Geometry: final body of the model. Coordinates: model frame, mm. Face numbers are marked on the shaded views. A direction names the side the tool comes from. Give positions to 0.01 mm unless a question says otherwise; leave off trailing zeros. Write each loop counter-clockwise with the first axis right and the second up, starting at its lowest first coordinate (ties: lowest second). Pieces come first, ordered by that corner, then holes. Notation, with made-up numbers: M 69.25,62 L 116.25,62 A30 cw 116.25,89 Z; hole C -21.5,39 d7. An arc over 180 degrees is marked long. Use one line per item in the form item = value. Start each with the question number.
Item 1: Pull-direction query (Y, two-part tool) for the marked faces 3, 4 and 5; classes: released by +Y, released by -Y, zero draft, split by the parting line, or undercut.
Item 2: Section query D-D on y = 507.5. Return loops of the section in (x, z), then the cut area to 3 significant figures.
Item 3: Section query A-A on z = -66.5. Return loops of the section in (x, y), then the cut area to 3 significant figures.
Item 4: Section query C-C on z = -90. Return loops of the section in (x, y), then the cut area to 3 significant figures.
Item 5: Contact query for flat-ended pins moving along their axis: P1, Ø2, axis at x = 14, z = -89, coming from the +Y side; P2, Ø6, axis at x = -17.5, z = -187.5, coming from the -Y side; P3, Ø3, axis at x = 18, z = -108, coming from the +Y side. Output: stop coordinate, or through.
Item 6: Material intervals for line 1 along Y through (x, z) = (5.5, -184.5); line 2 along Z through (x, y) = (12, 455.5); line 3 along Y through (x, z) = (-18, -91), sorted ascending. Write a range as from..to.
Item 7: Section query B-B on y = 456.5. Return loops of the section in (x, z).
Item 8: Access query for the marked faces 1 and 2. Directions: +Z, -Z, +X, -X, +Y, -Y. A direction counts if a zero-diameter tool reaches every point of the face in a straight line with its end or side. Return the directions, or none.
from build123d import *

# Parameters (mm, degrees)
BOSS_EXTRUDE1_DEPTH      = 12.238736
BOSS_EXTRUDE1_DEPTH_BACK = 12.238736
BOSS_EXTRUDE2_DEPTH      = 19.311112
BOSS_EXTRUDE2_DEPTH_BACK = 19.311112
BOSS_EXTRUDE3_DEPTH      = 20.236688
BOSS_EXTRUDE3_DEPTH_BACK = 20.236688
SKETCH3_R                = 29.891166833
BOSS_EXTRUDE4_DEPTH      = 36.886896
BOSS_EXTRUDE4_DEPTH_BACK = 36.886896
SKETCH4_R                = 19.656137362
SKETCH5_R                = 26.05024
CUT_EXTRUDE1_DEPTH       = 601.022741268
CHAMFER1_SIZE            = 1.66497
CHAMFER2_SIZE            = 2.486914


with BuildPart() as part:
    # Sketch1 → Boss-Extrude1 (new, two sides: drawn at the far end of the back side and taken through both)
    with BuildSketch(Plane(origin=(0, 0, 0), x_dir=(0, 0, -1), z_dir=(1, 0, 0)).offset(-BOSS_EXTRUDE1_DEPTH_BACK)):
        Polygon((177.038508, 548.169846), (190.081662, 534.280364), (128.192022, 468.216234), (114.7191, 481.689156), align=None)
    extrude(amount=BOSS_EXTRUDE1_DEPTH + BOSS_EXTRUDE1_DEPTH_BACK)

    # Sketch2 → Boss-Extrude2 (add, two sides: drawn at the far end of the back side and taken through both)
    with BuildSketch(Plane(origin=(0, 0, 0), x_dir=(0, 0, -1), z_dir=(1, 0, 0)).offset(-BOSS_EXTRUDE2_DEPTH_BACK)):
        Polygon((123.984766, 497.124482), (144.41805, 477.32315), (97.590864, 427.107096), (77.789786, 447.540126), align=None)
    extrude(amount=BOSS_EXTRUDE2_DEPTH + BOSS_EXTRUDE2_DEPTH_BACK)

    # Sketch3 → Boss-Extrude3 (add, two sides: drawn at the far end of the back side and taken through both)
    with BuildSketch(Plane(origin=(0, 0, 0), x_dir=(0, 0, -1), z_dir=(1, 0, 0)).offset(-BOSS_EXTRUDE3_DEPTH_BACK)):
        with Locations((86.798404, 438.166256)):
            Circle(SKETCH3_R)
    extrude(amount=BOSS_EXTRUDE3_DEPTH + BOSS_EXTRUDE3_DEPTH_BACK)

    # Sketch4 → Boss-Extrude4 (add, two sides: drawn at the far end of the back side and taken through both)
    with BuildSketch(Plane(origin=(0, 0, 0), x_dir=(0, 0, -1), z_dir=(1, 0, 0)).offset(-BOSS_EXTRUDE4_DEPTH_BACK)):
        with Locations((185.811668, 541.18891)):
            Circle(SKETCH4_R)
    extrude(amount=BOSS_EXTRUDE4_DEPTH + BOSS_EXTRUDE4_DEPTH_BACK)

    # Sketch5 → Cut-Extrude1 (cut, through all)
    with BuildSketch(Plane(origin=(20.236688, 0, 0), x_dir=(0, 0, -1), z_dir=(1, 0, 0))):
        with Locations((86.798404, 438.166256)):
            Circle(SKETCH5_R)
    extrude(amount=-CUT_EXTRUDE1_DEPTH, mode=Mode.SUBTRACT)

    # Chamfer1
    chamfer1_edges = [part.edges().sort_by_distance(p)[0] for p in [
        (12.238736, 501.953153429, -159.79715777),
        (-12.238736, 501.953153429, -159.79715777),
        (12.238736, 515.758092022, -146.655530324),
        (-12.238736, 515.758092022, -146.655530324),
    ]]
    chamfer(chamfer1_edges, length=CHAMFER1_SIZE)

    # Chamfer2
    chamfer2_edges = [part.edges().sort_by_distance(p)[0] for p in [
        (-19.311112, 481.919947716, -109.819549109),
        (19.311112, 481.919947716, -109.819549109),
        (19.311112, 461.841632324, -129.981314135),
        (-19.311112, 461.841632324, -129.981314135),
    ]]
    chamfer(chamfer2_edges, length=CHAMFER2_SIZE)


solid = part.part
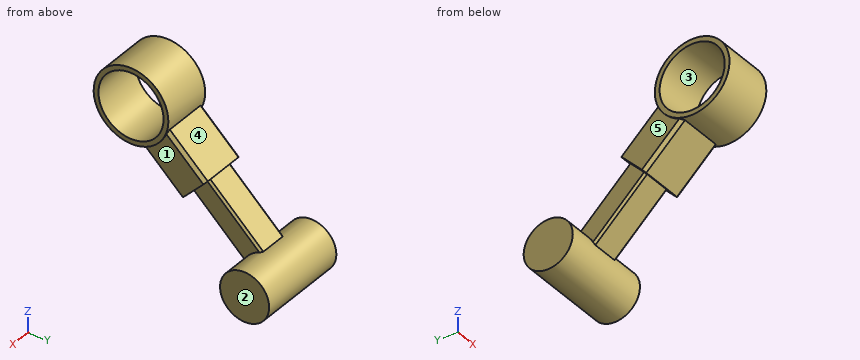
Answer sheet:
q1.face_3 = undercut
q1.face_4 = released by +Y
q1.face_5 = zero draft
q2.outline = M -12.24,-162.71 L -10.57,-164.99 L 10.57,-164.99 L 12.24,-162.71 L 12.24,-141.2 L 10.57,-138.91 L -10.57,-138.91 L -12.24,-141.2 Z
q2.area = 631 mm2
q3.outline = M -20.24,416.22 L 20.24,416.22 L 20.24,421.84 L -20.24,421.84 Z; M -20.24,454.49 L 20.24,454.49 L 20.24,460.11 L -20.24,460.11 Z
q3.area = 454 mm2
q4.outline = M -20.24,408.45 L 20.24,408.45 L 20.24,412.31 L -20.24,412.31 Z; M -20.24,464.02 L 20.24,464.02 L 20.24,467.89 L -20.24,467.89 Z
q4.area = 313 mm2
q5.P1 = 468.03
q5.P2 = 521.53
q5.P3 = 480.97
q6.line_1 = 521.58..560.8
q6.line_2 = -124.07..-106.24, -67.35..-62.45
q6.line_3 = 408.57..412.46, 463.88..467.76
q7.outline = M -20.24,-110.41 L -19.31,-110.41 L -19.31,-121.6 L -16.82,-125 L 16.82,-125 L 19.31,-121.6 L 19.31,-110.41 L 20.24,-110.41 L 20.24,-105.3 L -20.24,-105.3 Z; M -20.24,-68.29 L 20.24,-68.29 L 20.24,-63.19 L -20.24,-63.19 Z
q8.face_1 = -Z, +X, +Y
q8.face_2 = +Z, -Z, +X, +Y, -Y
